Build history of the part. All positions in model axes, mm. A direction names the side the tool comes from. Round coordinates to 2 decimals unless told otherwise and drop trailing zeros. Loops run counter-clockwise (first coordinate to the right, second up) from the corner with the lowest first, then second, coordinate; pieces in that order, holes last.
from build123d import *
from OCP.BRepFilletAPI import BRepFilletAPI_MakeChamfer

# Parameters (mm, degrees)
SKETCH_1_W          = 19.6
SKETCH_1_H          = 8
EXTRUDE_1_DEPTH     = 12.9
SKETCH_2_W          = 27.6
SKETCH_2_H          = 8
SKETCH_2_R          = 1
EXTRUDE_2_DEPTH     = 0.5
SKETCH_3_W          = 19.6
SKETCH_3_H          = 8
EXTRUDE_3_DEPTH     = 17.4
SKETCH_4_W          = 10
SKETCH_4_H          = 8
EXTRUDE_5_DEPTH     = 20
SKETCH_6_R          = 1.8
EXTRUDE_6_DEPTH     = 3
CUT_EXTRUDE_2_DEPTH = 17
CHAMFER_1_SIZE      = 0.3
CHAMFER_1_SIZE2     = 0.270121213


with BuildPart() as part:
    # 草图1 → 凸台-拉伸1 (new body)
    with BuildSketch(Plane(origin=(0, 0, 0), x_dir=(1, 0, 0), z_dir=(0, 1, 0))):
        Rectangle(SKETCH_1_W, SKETCH_1_H)
    extrude(amount=EXTRUDE_1_DEPTH)

    # 草图2 → 凸台-拉伸2 (add)
    with BuildSketch(Plane(origin=(0, 12.9, 0), x_dir=(1, 0, 0), z_dir=(0, 1, 0))):
        Rectangle(SKETCH_2_W, SKETCH_2_H)
        with Locations(Location((-11.8, 0, 0), (0, 0, 270))):
            Circle(SKETCH_2_R, mode=Mode.SUBTRACT)
        with Locations(Location((11.8, 0, 0), (0, 0, 270))):
            Circle(SKETCH_2_R, mode=Mode.SUBTRACT)
    extrude(amount=EXTRUDE_2_DEPTH)

    # 草图3 → 凸台-拉伸3 (add)
    with BuildSketch(Plane.XZ):
        Rectangle(SKETCH_3_W, SKETCH_3_H)
    extrude(amount=-EXTRUDE_3_DEPTH)

    # 草图4 → 凸台-拉伸5 (add)
    with BuildSketch(Plane(origin=(0, 0, 0), x_dir=(1, 0, 0), z_dir=(0, 1, 0))):
        with Locations((-4.8, 0)):
            Rectangle(SKETCH_4_W, SKETCH_4_H)
    extrude(amount=EXTRUDE_5_DEPTH)

    # 草图6 → 凸台-拉伸6 (add)
    with BuildSketch(Plane(origin=(0, 20, 0), x_dir=(1, 0, 0), z_dir=(0, 1, 0))):
        with Locations(Location((-5.8, 0, 0), (0, 0, 90))):
            Circle(SKETCH_6_R)
    extrude(amount=EXTRUDE_6_DEPTH)

    # 草图7 → 切除-拉伸2 (cut)
    with BuildSketch(Plane.XZ):
        with BuildLine():
            Line((14.367004184, -5.785535706), (9.389835398, -5.785535706))
            ThreePointArc((9.389835398, -5.785535706), (13.783545245, -0.444056645), (10.226439047, 5.487476064))
            Line((10.226439047, 5.487476064), (14.54010062, 5.487476064))
            Line((14.54010062, 5.487476064), (14.367004184, -5.785535706))
        make_face()
        with BuildLine():
            Line((-10.226439047, 5.487476064), (-14.54010062, 5.487476064))
            Line((-14.54010062, 5.487476064), (-14.367004184, -5.785535706))
            Line((-14.367004184, -5.785535706), (-9.389835398, -5.785535706))
            ThreePointArc((-9.389835398, -5.785535706), (-13.783545245, -0.444056645), (-10.226439047, 5.487476064))
        make_face()
    extrude(amount=-CUT_EXTRUDE_2_DEPTH, mode=Mode.SUBTRACT)

    # 倒角1: one chamfer whose edges measure the first distance from different faces: ONE call of the kernel's chamfer builder (chamfer() names one face for all edges)
    chamfer_1_edges_1 = [part.edges().sort_by_distance(p)[0] for p in [
        (9.8, 15.4, -4),
        (-9.8, 16.7, -4),
        (-4.8, 20, -4),
    ]]
    chamfer_1_side_1 = [part.faces().sort_by_distance(p)[0] for p in [
        (-0.337742628, 9.433402177, -4),
    ]]
    chamfer_1_edges_2 = [part.edges().sort_by_distance(p)[0] for p in [
        (-9.8, 16.7, 4),
        (5, 17.4, 4),
        (9.8, 15.4, 4),
        (0.2, 18.7, 4),
        (-4.8, 20, 4),
    ]]
    chamfer_1_side_2 = [part.faces().sort_by_distance(p)[0] for p in [
        (-0.337742628, 9.433402177, 4),
    ]]
    chamfer_1_edges_3 = [part.edges().sort_by_distance(p)[0] for p in [
        (9.8, 17.4, 0),
        (5, 17.4, -4),
    ]]
    chamfer_1_side_3 = [part.faces().sort_by_distance(p)[0] for p in [
        (5, 17.4, 0),
    ]]
    chamfer_1_edges_4 = [part.edges().sort_by_distance(p)[0] for p in [
        (0, 0, 4),
        (-9.8, 0, 0),
        (0, 0, -4),
    ]]
    chamfer_1_side_4 = [part.faces().sort_by_distance(p)[0] for p in [
        (0, 0, 0),
    ]]
    chamfer_1_edges_5 = [part.edges().sort_by_distance(p)[0] for p in [
        (0.2, 18.7, -4),
        (0.2, 20, 0),
    ]]
    chamfer_1_side_5 = [part.faces().sort_by_distance(p)[0] for p in [
        (0.2, 18.7, 0),
    ]]
    chamfer_1_edges_6 = [part.edges().sort_by_distance(p)[0] for p in [
        (9.8, 0, 0),
        (9.8, 6.45, 4),
        (9.8, 6.45, -4),
    ]]
    chamfer_1_side_6 = [part.faces().sort_by_distance(p)[0] for p in [
        (9.8, 6.45, 0),
    ]]
    chamfer_1_edges_7 = [part.edges().sort_by_distance(p)[0] for p in [
        (-9.8, 20, 0),
    ]]
    chamfer_1_side_7 = [part.faces().sort_by_distance(p)[0] for p in [
        (-9.8, 16.7, 0),
    ]]
    chamfer_1_edges_8 = [part.edges().sort_by_distance(p)[0] for p in [
        (-9.8, 6.45, 4),
        (-9.8, 6.45, -4),
    ]]
    chamfer_1_side_8 = [part.faces().sort_by_distance(p)[0] for p in [
        (-9.8, 6.45, 0),
    ]]
    chamfer_1 = BRepFilletAPI_MakeChamfer(part.part.solid().wrapped)
    for e in chamfer_1_edges_1:
        chamfer_1.Add(CHAMFER_1_SIZE, CHAMFER_1_SIZE2, e.wrapped, chamfer_1_side_1[0].wrapped)  # the first distance lies on this face
    for e in chamfer_1_edges_2:
        chamfer_1.Add(CHAMFER_1_SIZE, CHAMFER_1_SIZE2, e.wrapped, chamfer_1_side_2[0].wrapped)  # the first distance lies on this face
    for e in chamfer_1_edges_3:
        chamfer_1.Add(CHAMFER_1_SIZE, CHAMFER_1_SIZE2, e.wrapped, chamfer_1_side_3[0].wrapped)  # the first distance lies on this face
    for e in chamfer_1_edges_4:
        chamfer_1.Add(CHAMFER_1_SIZE, CHAMFER_1_SIZE2, e.wrapped, chamfer_1_side_4[0].wrapped)  # the first distance lies on this face
    for e in chamfer_1_edges_5:
        chamfer_1.Add(CHAMFER_1_SIZE, CHAMFER_1_SIZE2, e.wrapped, chamfer_1_side_5[0].wrapped)  # the first distance lies on this face
    for e in chamfer_1_edges_6:
        chamfer_1.Add(CHAMFER_1_SIZE, CHAMFER_1_SIZE2, e.wrapped, chamfer_1_side_6[0].wrapped)  # the first distance lies on this face
    for e in chamfer_1_edges_7:
        chamfer_1.Add(CHAMFER_1_SIZE, CHAMFER_1_SIZE2, e.wrapped, chamfer_1_side_7[0].wrapped)  # the first distance lies on this face
    for e in chamfer_1_edges_8:
        chamfer_1.Add(CHAMFER_1_SIZE, CHAMFER_1_SIZE2, e.wrapped, chamfer_1_side_8[0].wrapped)  # the first distance lies on this face
    add(Compound.cast(chamfer_1.Shape()), mode=Mode.REPLACE)


solid = part.part
(1) Probe line 1 (X direction, y = 13.05, z = 0); line 2 (Y direction, x = -2, z = -1.75); line 3 (X direction, y = 8, z = 0). List the from-to ranges inside material, lowest first.
Responses:
line 1: x = -13.8 to -12.8, -10.8 to 10.8, 12.8 to 13.8
line 2: y = 0 to 20
line 3: x = -9.8 to 9.8
(2) Pull direction Z, two halves, no side cores. Call faces 1 (the face through (-10.81, 13.15, -0.13)), 2 (the face through (-11, 13.4, 1)), 3 (the face through (-4, 21, 0)), 4 (the face through (10.824, 13.146, -0.217)): +Z half, -Z half, draft (parallel to the pull), parting line (faces both ways), or undercut.
Responses:
face 1: undercut
face 2: draft
face 3: parting line
face 4: undercut
(3) Slice it at D-D on y = 5.5. List the corners of the cut face in (x, z), plus the area to 3 significant figures.
Responses:
outline: (-9.8, -3.7) - (-9.53, -4) - (9.53, -4) - (9.8, -3.7) - (9.8, 3.7) - (9.53, 4) - (-9.53, 4) - (-9.8, 3.7) - close
area: 157 mm2
(4) Slice it at A-A on x = 11.8. List the corners of the cut face in (y, z), plus the area to 3 significant figures.
Responses:
outline: (12.9, -4) - (13.4, -4) - (13.4, -1) - (12.9, -1) - close; (12.9, 1) - (13.4, 1) - (13.4, 4) - (12.9, 4) - close
area: 3.00 mm2
(5) Slice it at B-B on z = 0. Count the separate pieces of the cut face and the enclosed holes in it, plus the area to 3 significant figures.
Responses:
separate pieces: 3
enclosed holes: 0
area: 380 mm2
(6) Pin check, flat tips, straight feed: P1, Ø2, axis at y = 6.5, z = -0.5, coming from the -X side; P2, Ø1, axis at y = 16.5, z = -2.5, coming from the +X side; P3, Ø2.5, axis at y = 19, z = -0.5, coming from the +X side; P4, Ø1.2, axis at x = -11.8, z = 0, coming from the +Y side. Stop position of each tip, or through.
Responses:
P1: stops at x = -9.8
P2: stops at x = 9.8
P3: stops at x = 0.2
P4: passes through
(7) Which spindle directions (+Z, -Z, +X, -X, +Y, -Y) get a long thin tool onto all of the face, cutting with end or side? Do faces 5 (the face through (-9.8, 6, 0)), 6 (the face through (0.2, 19, 0)), 7 (the face through (-9.8, 17, 0)). Say none if no direction does.
Responses:
face 5: +Z, -Z, -X, -Y
face 6: +Z, -Z, +X, +Y
face 7: +Z, -Z, -X, +Y
(8) Slice it at C-C on x = 7.25. List the corners of the cut face in (y, z).
Responses:
outline: (0, -3.7) - (0.27, -4) - (17.13, -4) - (17.4, -3.7) - (17.4, 3.73) - (17.1, 4) - (0.27, 4) - (0, 3.7) - close
